The model under review builds one solid part; all positions refer to its coordinate system, in mm. A direction names the side the tool comes from. Round coordinates to 2 decimals unless told otherwise and drop trailing zeros. Loops run counter-clockwise (first coordinate to the right, second up) from the corner with the lowest first, then second, coordinate; pieces in that order, holes last. Notation, with made-up numbers: M 21,85 L 73,85 A17 ccw 73,100 Z; hole C -9,2 d6. An arc over 180 degrees is marked long. Return JSON: item names as keys, results as strings. Group by question number.
Q1. For faces 1 (the face through (-22.647, -0.2, 24.5)), 2 (the face through (19.4, -14.43, 12.41)), 3 (the face through (18.4, -13.43, 12.68)), 4 (the face through (-21.221, -15.634, 24.493)), list the 3-axis set-ups (+Z, -Z, +X, -X, +Y, -Y) from which the entire face can be reached by the end or side of a thin tool; tool diameter is ignored.
Q2. Consider section C-C (x = 2.5). State the section outline as (y, z) points, and give its area (3 significant figures).
Q3. Consider section A-A (y = -8.5). State the section outline as (x, z) points, and give its area (3 significant figures).
Q4. Consider section B-B (z = 11.75). State the section outline as (x, y) points.
Q5. Clearance check with flat-ended pins moving along their axes: pin 1 Ø4 at (x, z) = (10.5, 11) entering from -Y; pin 2 Ø8 at (x, z) = (-6.5, 14.5) entering from +Y; pin 3 Ø0.8 at (x, z) = (-7, 24.5) entering from +Y. State where each tip first meets the part, or that it passes through.
Q6. To check wall thickness, follow line 1 along Y through (x, z) = (10.5, 14.25); line 2 along X through (y, z) = (-2.5, 14); line 3 along X through (y, z) = (-12.5, 1). State the ranges of each line that lie inside material, in increasing order.
Q7. Draft analysis for pull direction Z (two halves, no side actions). For faces 5 (the face through (-19.43, -14.4, 12.41)), 6 (the face through (0, -15, 25)), 7 (the face through (-20, 0, 12)), 8 (the face through (-21.221, 15.634, 24.493)), state which applies: pulls with the +Z half, pulls with the -Z half, needs draft (parallel to the pull), parting line crosses it, or undercut.
from build123d import *

# Parameters (mm, degrees)
F0_W     = 40
F0_H     = 30
F0_W_2   = 38
F0_H_2   = 28
F1_DEPTH = 25
F2_R     = 2
F3_W     = 45.2934801579
F3_H     = 34.2747867107
F3_W_2   = 38.8284271247
F3_H_2   = 28.8284271247
F4_DEPTH = 1
F5_R     = 5
F6_W     = 45.6778518856
F6_H     = 34.5805324614
F6_W_2   = 38
F6_H_2   = 28.8284271247
F7_DEPTH = 0.5
F8_R     = 5


with BuildPart() as f1:
    # F0 (on Top) → F1 (new body)
    with BuildSketch(Plane.XY):
        Rectangle(F0_W, F0_H)
        Rectangle(F0_W_2, F0_H_2, mode=Mode.SUBTRACT)
    extrude(amount=F1_DEPTH)

    # F2
    f2_edges = [f1.edges().sort_by_distance(p)[0] for p in [
        (-19, -14, 12.5),
        (-20, -15, 12.5),
        (-20, 15, 12.5),
        (-19, 14, 12.5),
        (19, -14, 12.5),
        (19, 14, 12.5),
        (20, 15, 12.5),
        (20, -15, 12.5),
    ]]
    fillet(f2_edges, radius=F2_R)

    # F3 (on face) → F4 (join)
    with BuildSketch(Plane.XY.offset(25)):
        Rectangle(F3_W, F3_H)
        Rectangle(F3_W_2, F3_H_2, mode=Mode.SUBTRACT)
    extrude(amount=-F4_DEPTH)

    # F5
    f5_edges = [f1.edges().sort_by_distance(p)[0] for p in [
        (-22.64674, 17.137393, 24.5),
        (-22.64674, -17.137393, 24.5),
        (22.64674, 17.137393, 24.5),
        (22.64674, -17.137393, 24.5),
    ]]
    fillet(f5_edges, radius=F5_R)

    # F6 (on face) → F7 (join, symmetric)
    with BuildSketch(Plane(origin=(0, 0, 0), x_dir=(1, 0, 0), z_dir=(0, 0, -1))):
        Rectangle(F6_W, F6_H)
        Rectangle(F6_W_2, F6_H_2, mode=Mode.SUBTRACT)
    extrude(amount=F7_DEPTH, both=True)

    # F8
    f8_edges = [f1.edges().sort_by_distance(p)[0] for p in [
        (-22.838926, -17.290266, 0),
        (22.838926, -17.290266, 0),
        (-22.838926, 17.290266, 0),
        (22.838926, 17.290266, 0),
    ]]
    fillet(f8_edges, radius=F8_R)


solid = f1.part
Values:
{
 "1": {"face 1": "+Z, -X, +Y, -Y", "face 2": "+X, -Y", "face 3": "+Z, -Z", "face 4": "+Z, -X, -Y"},
 "2": {"outline": "M -17.29,-0.5 L -14.41,-0.5 L -14.41,0 L -14,0 L -14,25 L -17.14,25 L -17.14,24 L -15,24 L -15,0.5 L -17.29,0.5 Z; M 14,0 L 14.41,0 L 14.41,-0.5 L 17.29,-0.5 L 17.29,0.5 L 15,0.5 L 15,24 L 17.14,24 L 17.14,25 L 14,25 Z", "area": "59.4 mm2"},
 "3": {"outline": "M -22.84,-0.5 L -19,-0.5 L -19,25 L -22.65,25 L -22.65,24 L -20,24 L -20,0.5 L -22.84,0.5 Z; M 19,-0.5 L 22.84,-0.5 L 22.84,0.5 L 20,0.5 L 20,24 L 22.65,24 L 22.65,25 L 19,25 Z", "area": "62.0 mm2"},
 "4": {"outline": "M -20,-13 A2 ccw -18,-15 L 18,-15 A2 ccw 20,-13 L 20,13 A2 ccw 18,15 L -18,15 A2 ccw -20,13 Z; hole M -19,-12 A2 ccw -17,-14 L 17,-14 A2 ccw 19,-12 L 19,12 A2 ccw 17,14 L -17,14 A2 ccw -19,12 Z"},
 "5": {"pin 1": "stops at y = -15", "pin 2": "stops at y = 15", "pin 3": "stops at y = 17.14"},
 "6": {"line 1": "y = -15 to -14, 14 to 15", "line 2": "x = -20 to -19, 19 to 20", "line 3": "x = -20 to -18.94, 18.94 to 20"},
 "7": {"face 5": "undercut", "face 6": "pulls with the +Z half", "face 7": "undercut", "face 8": "needs draft"}
}
